Can you work these out from the model? Positions are in its coordinate system, mm. Face numbers are marked on the shaded views. A direction names the side the tool comes from. Give positions to 0.01 mm unless a question says otherwise; leave off trailing zeros. Write each loop counter-clockwise with the first axis right and the second up, starting at its lowest first coordinate (ties: lowest second). Pieces come first, ordered by that corner, then holes. Notation, with made-up numbers: (35, -4.75) - (93, -4.75) arc R20 ccw to (93, 24.25) - close; hole circle Ø8 at (-21.5, 56.5). An arc over 180 degrees is marked (long way). Return JSON: item names as keys, results as strings. Group by question number.
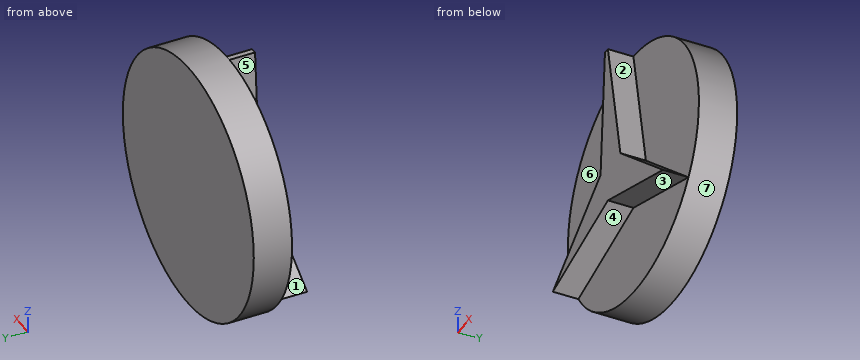
from build123d import *

# Parameters (mm, degrees)
F1_DEPTH = 12.7
F2_R     = 25.4
F3_DEPTH = 7.62


with BuildPart() as f1:
    # F0 (on Front) → F1 (new body)
    with BuildSketch(Plane.XZ):
        Polygon((0, 25.373987), (-1.149251, 25.373987), (-2.861024, 0), (-21.364293, -13.737794), (0, -7.201886), (21.364293, -13.737794), (4.834144, 0), align=None)
    extrude(amount=F1_DEPTH)

    # F2 (on Front) → F3 (join)
    with BuildSketch(Plane.XZ):
        Circle(F2_R)
    extrude(amount=F3_DEPTH)


solid = f1.part
1) I need wall thicknesses on line 1 along Y through (x, z) = (-22, 5); line 2 along X through (y, z) = (-10.5, 9.5); line 3 along Z through (x, y) = (-13, -11.5). Which ranges of each line are inside material? Lowest first, please.
2) Imagine slicing it at B-B, the plane x = -12.5. Write out the boundary of the cut face in (y, z).
3) Will these pins go through, and if not, where does the flat tip stop? pin 1 Ø4 at (x, y) = (14, -5.5) entering from -Z; pin 2 Ø5.5 at (x, z) = (-1, -19) entering from -Y; pin 3 Ø2 at (y, z) = (-6.5, -5) entering from +X.
4) Imagine slicing it at A-A, the plane y = -9. Write out the boundary of the cut face in (x, z), and give its area (3 significant figures).
5) We'd pull the mould along X, two halves only. Please class the marked faces 4, 5, 6 and 7: pulls with the +X half, pulls with the -X half, needs draft (parallel to the pull), parting line crosses it, or undercut.
6) Imagine slicing it at D-D, the plane y = -1.5. Write out the boundary of the cut face in (x, z).
7) Imagine slicing it at C-C, the plane z = 21.5. Write out the boundary of the cut face in (x, y), and give its area (3 significant figures).
8) On a 3-axis mill with a long thin cutter (end or side, diameter ignored), from which of +Z, -Z, +X, -X, +Y, -Y can I reach the whole of each face in a straight line? I mean the marked faces 1, 2 and 3. Say none if no direction works.
Resolved:
{
 "1": {"line 1": "-7.62 to 0", "line 2": "-2.22 to 3.02", "line 3": "-11.18 to -7.53"},
 "2": {"outline": "(-12.7, -11.03) - (-7.62, -11.03) - (-7.62, -22.11) - (0, -22.11) - (0, 22.11) - (-7.62, 22.11) - (-7.62, -7.16) - (-12.7, -7.16) - close"},
 "3": {"pin 1": "z = -22.39", "pin 2": "y = -7.62", "pin 3": "x = 25.08"},
 "4": {"outline": "(-21.36, -13.74) - (0, -7.2) - (21.36, -13.74) - (4.83, 0) - (0, 25.37) - (-1.15, 25.37) - (-2.86, 0) - close", "area": "319 mm^2"},
 "5": {"face 4": "undercut", "face 5": "pulls with the -X half", "face 6": "needs draft", "face 7": "parting line crosses it"},
 "6": {"outline": "circle Ø50.8 at (0, 0)"},
 "7": {"outline": "(-13.52, -7.62) - (-1.41, -7.62) - (-1.41, -12.7) - (0.74, -12.7) - (0.74, -7.62) - (13.52, -7.62) - (13.52, 0) - (-13.52, 0) - close", "area": "217 mm^2"},
 "8": {"face 1": "+Z, -X, -Y", "face 2": "+Z, +X, -Y", "face 3": "-Z, -Y"}
}
